For this review, use the dimensioned drawing (mm, ordinates from the lowest corner) and the shaded views. Round coordinates to 2 decimals unless told otherwise and drop trailing zeros. Write each loop counter-clockwise with the first axis right and the second up, starting at its lowest first coordinate (ties: lowest second). Pieces come first, ordered by that corner, then holes. Notation, with made-up numbers: M 60.25,-23 L 69.25,-23 A18 cw 69.25,10 Z; hole C 58,-30 d10. An arc over 180 degrees is marked long. One line per question, with ' | ' between items. Start each with the question number.
Item 1: Add section D-D, the plane z = 22.5. State the section outline as (x, y) points, and give its area (3 significant figures).
Item 2: Add section A-A, the plane x = 60. State the section outline as (y, z) points.
Item 3: Add section C-C, the plane y = 4.2. Give the number of separate pieces and of enclosed holes in the cut face, and give its area (3 significant figures).
Item 4: For L1, parallel to Z at x = 180, y = 2.15; L2, parallel to Z at x = 126.5, y = 3.1; L3, parallel to Z at x = 35, y = 3.15, list the stretches that pass through material, from the lowest coordinate up.
Item 5: Add section B-B, the plane z = 55. State the section outline as (x, y) points, and give its area (3 significant figures).
Item 6: Insertion check: pin 1 Ø7 at (x, z) = (15, 118) entering from -Y. The pin has a flat end and moves straight along its axis. Give the tip position at first contact, or say it passes through.
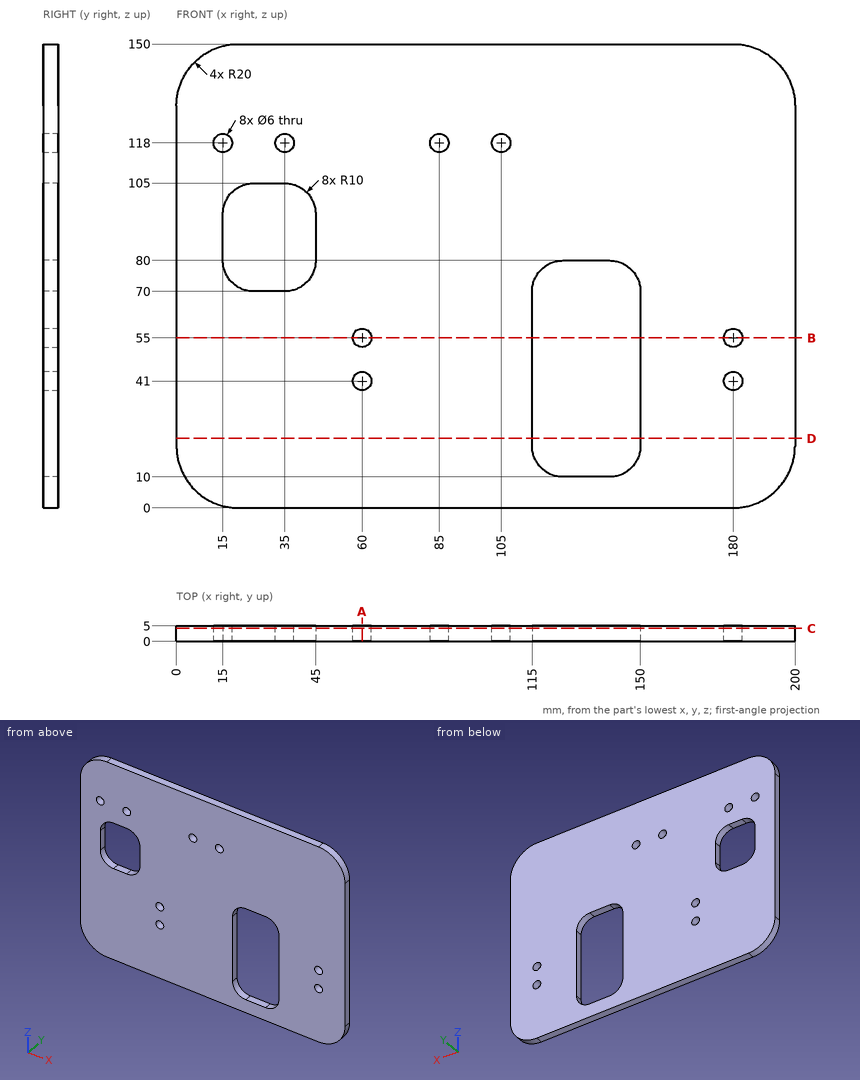
Computed values:
1) outline: M 0,0 L 115,0 L 115,5 L 0,5 Z; M 150,0 L 200,0 L 200,5 L 150,5 Z | area: 825 mm^2
2) outline: M 0,0 L 5,0 L 5,38 L 0,38 Z; M 0,44 L 5,44 L 5,52 L 0,52 Z; M 0,58 L 5,58 L 5,150 L 0,150 Z
3) separate pieces: 1 | enclosed holes: 10 | area: 26,100 mm^2
4) L1: z = 0 to 38, 44 to 52, 58 to 150 | L2: z = 0 to 10, 80 to 150 | L3: z = 0 to 70, 105 to 115, 121 to 150
5) outline: M 0,0 L 57,0 L 57,5 L 0,5 Z; M 63,0 L 115,0 L 115,5 L 63,5 Z; M 150,0 L 177,0 L 177,5 L 150,5 Z; M 183,0 L 200,0 L 200,5 L 183,5 Z | area: 765 mm^2
6) pin 1: stops at y = 0
